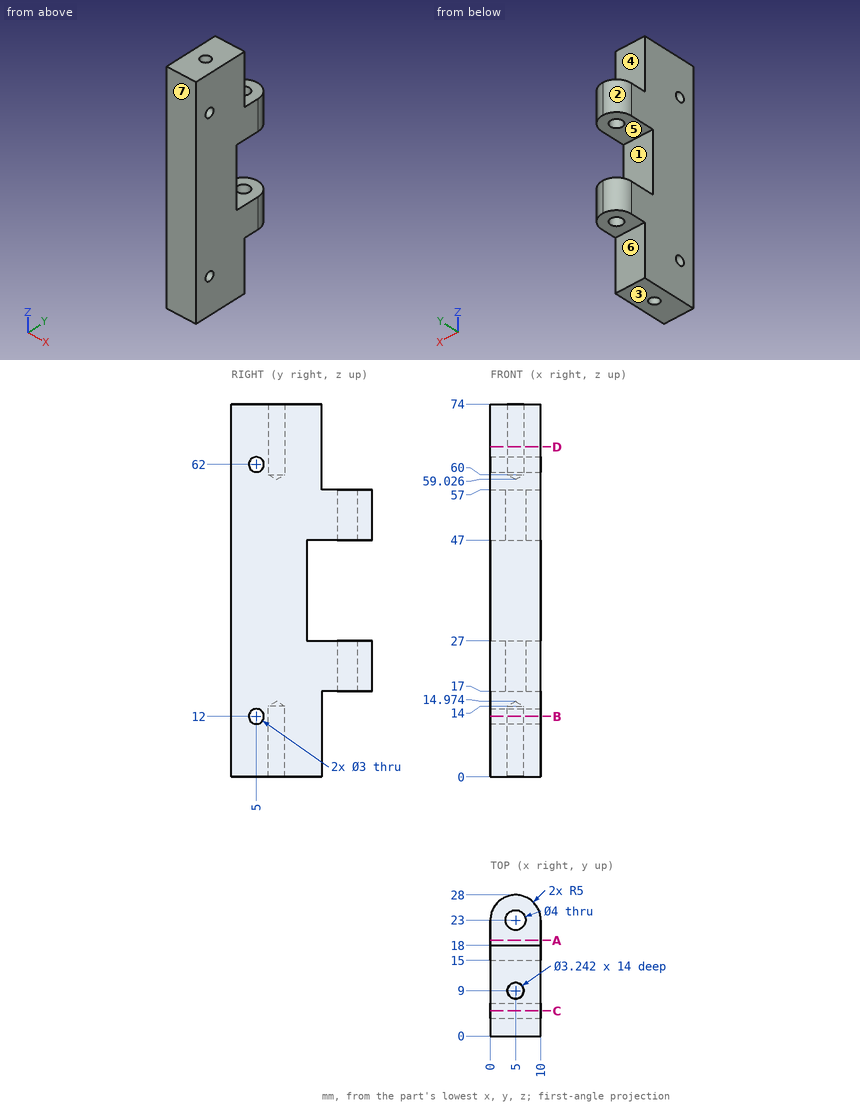
Part print with two shaded views. Sizes in mm from the minimum x, y, z corner. A direction names the side the tool comes from. Round coordinates to 2 decimals unless told otherwise and drop trailing zeros. Order: outer loops, then holes, each group sorted by start corner. A loop starts at its lowest first (then second) coordinate and runs counter-clockwise, first axis right, second up.
(1) Pin check, flat tips, straight feed: pin 1 (4.5 mm diameter, centred on x = 5, y = 23, fed in from -Z); pin 2 (3 mm diameter, centred on x = 5, z = 33, fed in from +Y); pin 3 (6 mm diameter, centred on y = 24.5, z = 15, fed in from -X); pin 4 (5 mm diameter, centred on x = 5, y = 23, fed in from +Z). Stop position of each tip, or through.
(2) Band-saw the part on D-D (z = 65.5). List the corners of the cut face in (x, y).
(3) Band-saw the part on B-B (z = 12). List the corners of the cut face in (x, y).
(4) Band-saw the part on A-A (y = 19). List the corners of the cut face in (x, z), then the cut area to 3 significant figures.
(5) 3-axis set-ups, long thin cutter, end or side, ignore diameter. For the marked faces 4, 5, 6 and 7: which of +Z, -Z, +X, -X, +Y, -Y reach the whole face in a straight line?
(6) Band-saw the part on C-C (y = 5). List the corners of the cut face in (x, z), then the cut area to 3 significant figures.
(7) Pull direction Z, two halves, no side cores. Call the marked faces 1, 2 and 3: released by +Z, released by -Z, zero draft, split by the parting line, or undercut.
(8) Drill centre lines: line 1 (Z direction, x = 5.5, y = 5); line 2 (Y direction, x = 5, z = 5.5); line 3 (Z direction, x = 5.75, y = 20). Where is each one in solid material? Low to high.
Verdict:
1. pin 1: stops at z = 17
1. pin 2: stops at y = 15
1. pin 3: stops at x = 0
1. pin 4: stops at z = 57
2. outline: (0, 0) - (10, 0) - (10, 18) - (0, 18) - close; hole circle Ø3.24 at (5, 9)
3. outline: (0, 0) - (10, 0) - (10, 3.5) - (0, 3.5) - close; (0, 6.5) - (10, 6.5) - (10, 18) - (0, 18) - close; hole circle Ø3.24 at (5, 9)
4. outline: (0, 17) - (10, 17) - (10, 27) - (0, 27) - close; (0, 47) - (10, 47) - (10, 57) - (0, 57) - close
4. area: 200 mm2
5. face 4: +Z, +X, -X, +Y
5. face 5: +X, -X, +Y
5. face 6: -Z, +X, -X, +Y
5. face 7: +Z, -Z, +X, -X, -Y
6. outline: (0, 0) - (10, 0) - (10, 10.5) - (0, 10.5) - close; (0, 13.5) - (10, 13.5) - (10, 60.5) - (0, 60.5) - close; (0, 63.5) - (10, 63.5) - (10, 74) - (0, 74) - close
6. area: 680 mm2
7. face 1: undercut
7. face 2: zero draft
7. face 3: released by -Z
8. line 1: z = 0 to 10.5, 13.5 to 60.5, 63.5 to 74
8. line 2: y = 0 to 7.38, 10.62 to 18
8. line 3: z = 17 to 27, 47 to 57
